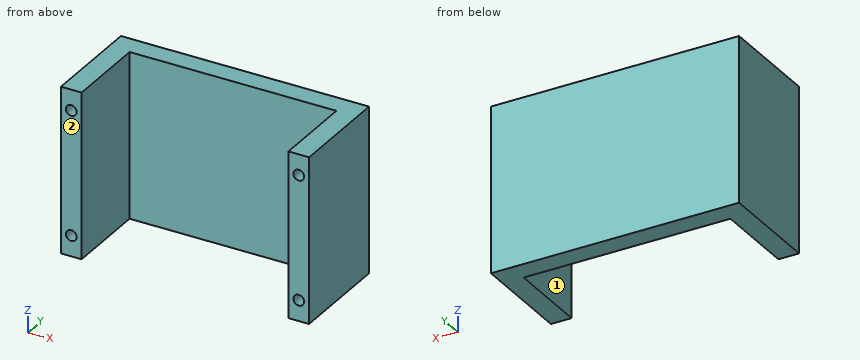
Autodesk Inventor part; units mm, degrees
ref_plane "YZ Plane" through (0, 0, 0) normal (1, 0, 0) x (0, 1, 0)
ref_plane "XZ Plane" through (0, 0, 0) normal (0, 1, 0) x (-1, 0, 0)
ref_plane "XY Plane" through (0, 0, 0) normal (0, 0, 1) x (1, 0, 0)
sketch "Sketch1" plane through (0, 0, 0) normal (0, 0, 1) x (1, 0, 0)
  line L0 (0, 0) -> (76.2, 0)
  line L1 (76.2, 0) -> (76.2, 31.75)
  line L2 (76.2, 31.75) -> (0, 31.75)
  line L3 (0, 31.75) -> (0, 0)
  line L4 (6.35, 0) -> (69.85, 0)
  line L5 (69.85, 0) -> (69.85, 25.4)
  line L6 (69.85, 25.4) -> (6.35, 25.4)
  line L7 (6.35, 25.4) -> (6.35, 0)
  dimension "d0" = 6.35
  dimension "d1" = 6.35
  dimension "d2" = 6.35
  dimension "d3" = 63.5
  dimension "d4" = 31.75
extrude "Extrusion1" add sketch "Sketch1" along normal blind 50.8 contours L3 L2 L1 L0 L5 L6 L7
sketch "Sketch2" plane through (0, 0, 0) normal (0, -1, 0) x (1, 0, 0)
  point P0 (0, 0)
ref_plane "Work Plane1" through (0, 0, 25.4) normal (0, 0, 1) x (1, 0, 0)
ref_plane "Work Plane2" through (38.1, 0, 0) normal (-1, 0, 0) x (0, 0, 1)
sketch "Sketch3" plane through (0, 0, 0) normal (0, -1, 0) x (1, 0, 0)
  circle A0 centre (3.175, 44.45) radius 1.651
  line L0 (0, 50.8) -> (6.35, 50.8)
  line L1 (6.35, 0) -> (6.35, 50.8)
  line L2 (0, 25.4) -> (76.2, 25.4)
  line L3 (76.2, 0) -> (76.2, 50.8)
  circle A1 centre (3.175, 6.35) radius 1.651
  line L4 (38.1, 50.8) -> (38.1, 0)
  circle A2 centre (73.025, 6.35) radius 1.651
  circle A3 centre (73.025, 44.45) radius 1.651
  point P0 (0, 0)
  dimension "d7" = 3.302
  dimension "d8" = 6.35
  dimension "d9" = 3.175
extrude "Extrusion2" cut sketch "Sketch3" against normal blind 12.7
properties part number "wirebridge2"
Part model, mm, in its own coordinate system. Face numbers are marked on the shaded views. A direction names the side the tool comes from. Give positions to 0.01 mm unless a question says otherwise; leave off trailing zeros. Order: outer loops, then holes, each group sorted by start corner. A loop starts at its lowest first (then second) coordinate and runs counter-clockwise, first axis right, second up. Notation, with made-up numbers: (55, 11.5) -> (102, 11.5) arc R24 ccw to (102, 40.5) -> close; hole circle Ø1 at (21, -33.75). An arc over 180 degrees is marked (long way). Use one line per item in the form item = value.
(1) Drill centre lines: line 1 (X direction, y = 24.5, z = 32); line 2 (X direction, y = 6, z = 6); line 3 (Y direction, x = 53, z = 24). Where is each one in solid material? Low to high. Write a range as from..to.
Solution:
line_1 = 0..6.35, 69.85..76.2
line_2 = 0..1.56, 4.79..6.35, 69.85..71.41, 74.64..76.2
line_3 = 25.4..31.75
(2) Saw through at C-C (z = 6.35). Write the cut outline in (x, y).
Solution:
outline = (0, 0) -> (1.52, 0) -> (1.52, 12.7) -> (4.83, 12.7) -> (4.83, 0) -> (6.35, 0) -> (6.35, 25.4) -> (69.85, 25.4) -> (69.85, 0) -> (71.37, 0) -> (71.37, 12.7) -> (74.68, 12.7) -> (74.68, 0) -> (76.2, 0) -> (76.2, 31.75) -> (0, 31.75) -> close
(3) Tool access for the marked faces 1 and 2: list every direction of +Z, -Z, +X, -X, +Y, -Y with a clear straight run to the whole face (end or side of a thin tool).
Solution:
face_1 = +Z, -Z, -Y
face_2 = +Z, -Z, +X, -X, -Y
(4) Saw through at B-B (y = 11). Write the cut outline in (x, z) (3 decimals).
Solution:
outline = (0, 0) -> (6.35, 0) -> (6.35, 50.8) -> (0, 50.8) -> close; (69.85, 0) -> (76.2, 0) -> (76.2, 50.8) -> (69.85, 50.8) -> close; hole circle Ø3.302 at (3.175, 6.35); hole circle Ø3.302 at (3.175, 44.45); hole circle Ø3.302 at (73.025, 6.35); hole circle Ø3.302 at (73.025, 44.45)
(5) Saw through at A-A (y = 15.5). Write the cut outline in (x, z).
Solution:
outline = (0, 0) -> (6.35, 0) -> (6.35, 50.8) -> (0, 50.8) -> close; (69.85, 0) -> (76.2, 0) -> (76.2, 50.8) -> (69.85, 50.8) -> close
(6) Flat gauge pins, fed straight in: P1, Ø1.5, axis at x = 65.5, z = 29, coming from the -Y side; P2, Ø1, axis at x = 73, z = 44.5, coming from the -Y side. Where does each tip first touch, or does it go through?
Solution:
P1 = 25.4
P2 = 12.7
(7) Saw through at D-D (x = 47.5). Write the cut outline in (y, z), then the cut area to 3 significant figures.
Solution:
outline = (25.4, 0) -> (31.75, 0) -> (31.75, 50.8) -> (25.4, 50.8) -> close
area = 323 mm²
